Can you work these out from the drawing? Everything is in mm from the part's minimum corner. A direction names the side the tool comes from. Give positions to 0.01 mm unless a question says otherwise; leave off trailing zeros. Write each loop counter-clockwise with the first axis right and the second up, starting at its lowest first coordinate (ties: lowest second). Pieces come first, ordered by that corner, then holes. Notation, with made-up numbers: (83, 23.5) -> (98, 23.5) arc R7 ccw to (98, 28.5) -> close; hole circle Ø8 at (-1.5, 10). An arc over 180 degrees is marked (long way). Use one line per item in the form item = value.
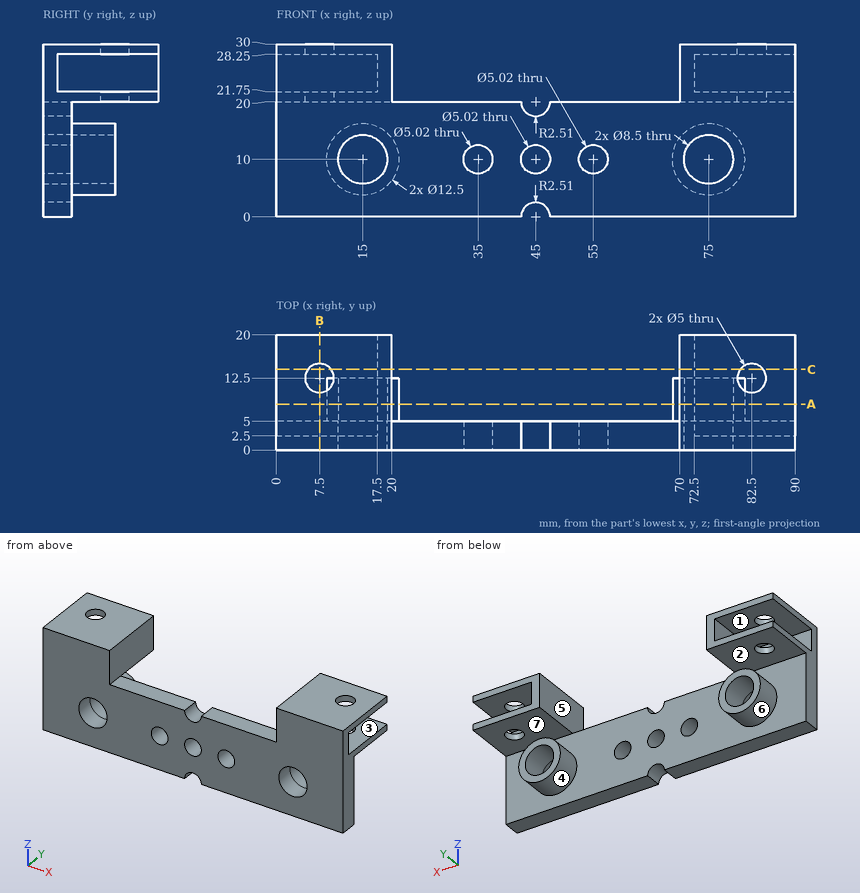
Q1. If I drill on line 1 along X through (y, z) = (1.45, 10); line 2 along Y through (x, z) = (82.5, 20.6); line 3 along X through (y, z) = (11.75, 27.25), over which ranges is the centre line in solid material (lowest first)? Write a range as from..to.
Result set:
line_1 = 0..10.75, 19.25..32.49, 37.51..42.49, 47.51..52.49, 57.51..70.75, 79.25..90
line_2 = 0..10, 15..20
line_3 = 17.5..20, 70..72.5
Q2. Which directions (+Z, -Z, +X, -X, +Y, -Y) give clear straight access to the entire face, cutting with the end or side of a thin tool? Please do the marked faces 1, 2, 3, 4 and 5.
Result set:
face_1 = -X, +Y
face_2 = +X, -X, +Y
face_3 = +X, +Y
face_4 = +Y
face_5 = +Z, +Y, -Y
Q3. I want a section at A-A, the plane y = 8. Write out the boundary of the cut face in (x, z).
Result set:
outline = (0, 20) -> (20, 20) -> (20, 30) -> (0, 30) -> (0, 28.25) -> (17.5, 28.25) -> (17.5, 21.75) -> (0, 21.75) -> close; circle Ø12.5 at (15, 10); circle Ø12.5 at (75, 10); (70, 20) -> (90, 20) -> (90, 21.75) -> (72.5, 21.75) -> (72.5, 28.25) -> (90, 28.25) -> (90, 30) -> (70, 30) -> close; hole circle Ø8.5 at (15, 10); hole circle Ø8.5 at (75, 10)
Q4. If we mould it in two halves opening along X, with no side actions, what happens to the marked faces 6 and 7? For each: +X half, -X half, draft (parallel to the pull), parting line (faces both ways), or undercut.
Result set:
face_6 = undercut
face_7 = draft
Q5. I want a section at B-B, the plane x = 7.5. Write out the boundary of the cut face in (y, z).
Result set:
outline = (0, 0) -> (5, 0) -> (5, 20) -> (10, 20) -> (10, 21.75) -> (2.5, 21.75) -> (2.5, 28.25) -> (10, 28.25) -> (10, 30) -> (0, 30) -> close; (15, 20) -> (20, 20) -> (20, 21.75) -> (15, 21.75) -> close; (15, 28.25) -> (20, 28.25) -> (20, 30) -> (15, 30) -> close
Q6. I want a section at C-C, the plane y = 14. Count the separate pieces of the cut face and the enclosed holes in it, and give its area (4 significant figures).
Result set:
separate_pieces = 6
enclosed_holes = 0
area = 144.5 mm2
Q7. Will these pins go through, and if not, where does the flat tip stop? pin 1 Ø3 at (x, z) = (13, 24.5) entering from +Y; pin 2 Ø8 at (x, y) = (66, 13.5) entering from -Z; pin 3 Ø6 at (x, y) = (7.5, 12.5) entering from -Z; pin 4 Ø6.5 at (x, y) = (82.5, 12.5) entering from +Z.
Result set:
pin_1 = 2.5
pin_2 = 6.43
pin_3 = 5.66
pin_4 = 30
